Input: part model. Units: mm. Frame: model coordinates. Face numbers are marked on the shaded views. A direction names the side the tool comes from. Round coordinates to 2 decimals unless told otherwise and drop trailing zeros. Loops run counter-clockwise (first coordinate to the right, second up) from the corner with the lowest first, then second, coordinate; pieces in that order, holes last. Notation, with made-up numbers: (-22.5, 40.5) -> (-10.5, 40.5) arc R32 ccw to (-10.5, 73.5) -> close; hole circle Ø9 at (-33, -9). An arc over 180 degrees is marked (long way). Answer as a JSON object with one key per item and string values. Group by question number.
Item 1: Section query B-B on x = 16. Return loops of the section in (y, z).
Item 2: Section query C-C on z = 70.5. Return loops of the section in (x, y), and give its area (3 significant figures).
Item 3: Section query A-A on y = -12. Return loops of the section in (x, z), and give its area (3 significant figures).
Item 4: Material intervals for line 1 (Z direction, x = -7.5, y = 5); line 2 (Y direction, x = 0, z = 71); line 3 (X direction, y = 0.5, z = 22), sorted ascending. Write a range as [from, to].
Item 5: Draft query along Z for the marked faces 1, 2 and 3. Return one class per face: released by +Z, released by -Z, zero draft, split by the parting line, or undercut.
Item 6: Pin query (flat end, axial travel): pin 1 (7.5 mm diameter, centred on x = 0, z = 12.7, fed in from +Y); pin 2 (4 mm diameter, centred on x = 0, z = 83.11, fed in from +Y); pin 3 (3 mm diameter, centred on y = 4.5, z = 15.5, fed in from +X); pin 4 (7.5 mm diameter, centred on x = 0, z = 64.06, fed in from -Y). Return the tip coordinate at first contact, or that it passes through.
Item 7: Set-up query: the marked faces 4, 5 and 6. Return all of +Z, -Z, +X, -X, +Y, -Y with unobstructed straight access to the full face (end or side cutting, diameter ignored); none if empty.
Item 8: Section query D-D on x = -4.5. Return loops of the section in (y, z), and give its area (3 significant figures).
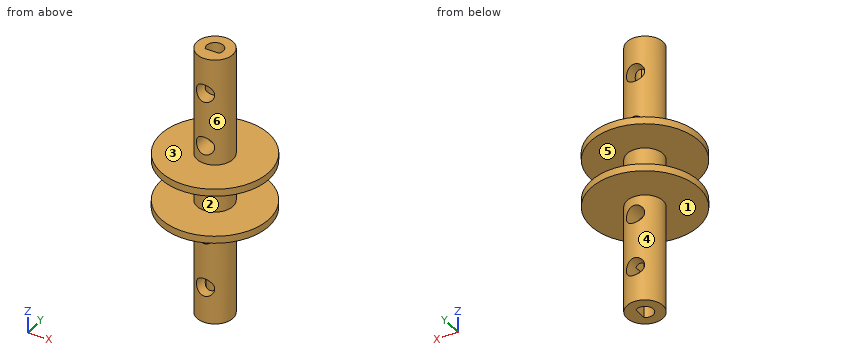
from build123d import *

# Parameters (mm, degrees)
SKETCH1_R               = 6.35
BOSS_EXTRUDE1_DEPTH     = 95.8088
SKETCH4_R               = 3.175
CUT_EXTRUDE2_DEPTH      = 7.35
CUT_EXTRUDE2_DEPTH_BACK = 7.35
SKETCH5_R               = 19.05
BOSS_EXTRUDE2_DEPTH     = 2.54
SKETCH6_R               = 19.05
BOSS_EXTRUDE3_DEPTH     = 2.54
CUT_EXTRUDE4_DEPTH      = 27.94
CUT_EXTRUDE5_DEPTH      = 27.94


with BuildPart() as part:
    # Sketch1 → Boss-Extrude1 (new body)
    with BuildSketch(Plane.XY):
        Circle(SKETCH1_R)
    extrude(amount=BOSS_EXTRUDE1_DEPTH)

    # Sketch4 → Cut-Extrude2 (cut, two sides)
    with BuildSketch(Plane(origin=(0, 0, 0), x_dir=(1, 0, 0), z_dir=(0, 1, 0))) as cut_extrude2_sk:
        with Locations((0, -83.1088)):
            Circle(SKETCH4_R)
        with Locations((0, -12.7)):
            Circle(SKETCH4_R)
        with Locations((0, -64.0588)):
            Circle(SKETCH4_R)
        with Locations((0, -31.75)):
            Circle(SKETCH4_R)
    extrude(amount=CUT_EXTRUDE2_DEPTH, mode=Mode.SUBTRACT)
    extrude(cut_extrude2_sk.sketch, amount=-CUT_EXTRUDE2_DEPTH_BACK, mode=Mode.SUBTRACT)

    # Sketch5 → Boss-Extrude2 (add)
    with BuildSketch(Plane.XY.offset(57.7088)):
        Circle(SKETCH5_R)
    extrude(amount=-BOSS_EXTRUDE2_DEPTH)

    # Sketch6 → Boss-Extrude3 (add)
    with BuildSketch(Plane(origin=(0, 0, 38.1), x_dir=(-1, 0, 0), z_dir=(0, 0, -1))):
        Circle(SKETCH6_R)
    extrude(amount=-BOSS_EXTRUDE3_DEPTH)

    # Sketch2 → Cut-Extrude4 (cut)
    with BuildSketch(Plane.XY.offset(95.8088)):
        with BuildLine():
            Line((-2.3368, -1.7526), (2.3368, -1.7526))
            ThreePointArc((2.3368, -1.7526), (0, 2.921), (-2.3368, -1.7526))
        make_face()
    extrude(amount=-CUT_EXTRUDE4_DEPTH, mode=Mode.SUBTRACT)

    # Sketch7 → Cut-Extrude5 (cut)
    with BuildSketch(Plane(origin=(0, 0, 0), x_dir=(-1, 0, 0), z_dir=(0, 0, -1))):
        with BuildLine():
            Line((-1.7526, 2.3368), (-1.7526, -2.3368))
            ThreePointArc((-1.7526, -2.3368), (1.306310912, -2.612621825), (2.921, 0))
            ThreePointArc((2.921, 0), (1.306310912, 2.612621825), (-1.7526, 2.3368))
        make_face()
    extrude(amount=-CUT_EXTRUDE5_DEPTH, mode=Mode.SUBTRACT)


solid = part.part
Solved:
{
 "1": {"outline": "(-10.34, 38.1) -> (10.34, 38.1) -> (10.34, 40.64) -> (-10.34, 40.64) -> close; (-10.34, 55.17) -> (10.34, 55.17) -> (10.34, 57.71) -> (-10.34, 57.71) -> close"},
 "2": {"outline": "circle Ø12.7 at (0, 0); hole (-2.34, -1.75) -> (2.34, -1.75) arc R2.92 ccw (long way) to start", "area": "104 mm²"},
 "3": {"outline": "(-14.8, 38.1) -> (14.8, 38.1) -> (14.8, 40.64) -> (-14.8, 40.64) -> close; (-14.8, 55.17) -> (14.8, 55.17) -> (14.8, 57.71) -> (-14.8, 57.71) -> close", "area": "150 mm²"},
 "4": {"line 1": "[38.1, 40.64], [55.17, 57.71]", "line 2": "[-6.35, -1.75], [2.92, 6.35]", "line 3": "[-6.33, -2.88], [1.75, 6.33]"},
 "5": {"face 1": "released by -Z", "face 2": "undercut", "face 3": "released by +Z"},
 "6": {"pin 1": "y = 6.35", "pin 2": "through", "pin 3": "x = 5.6", "pin 4": "y = -6.35"},
 "7": {"face 4": "-Z", "face 5": "none", "face 6": "+Z"},
 "8": {"outline": "(-18.51, 38.1) -> (-4.48, 38.1) -> (-4.48, 0) -> (4.48, 0) -> (4.48, 38.1) -> (18.51, 38.1) -> (18.51, 40.64) -> (4.48, 40.64) -> (4.48, 55.17) -> (18.51, 55.17) -> (18.51, 57.71) -> (4.48, 57.71) -> (4.48, 95.81) -> (-4.48, 95.81) -> (-4.48, 57.71) -> (-18.51, 57.71) -> (-18.51, 55.17) -> (-4.48, 55.17) -> (-4.48, 40.64) -> (-18.51, 40.64) -> close", "area": "1,000 mm²"}
}
